Here's how the part is built. I have some questions about the finished solid (model axes, mm). A direction names the side the tool comes from. Round coordinates to 2 decimals unless told otherwise and drop trailing zeros. Write each loop counter-clockwise with the first axis right and the second up, starting at its lowest first coordinate (ties: lowest second). Pieces come first, ordered by that corner, then holes. Notation, with made-up numbers: (-19, -1.5) - (38, -1.5) arc R5 ccw to (38, 6.5) - close; hole circle Ø4 at (-4.75, 65.25). An arc over 180 degrees is marked (long way). Use one line per item in the form item = value. Start each with the question number.
1. I want a section at D-D, the plane z = 6. List the corners of the cut face in (x, y) for me, plus the area to 3 significant figures.
2. Which directions (+Z, -Z, +X, -X, +Y, -Y) give clear straight access to the entire face, cutting with the end or side of a thin tool? Please do faces 1 (the flat face through (-9, 0, 6)), 2 (the cylindrical face through (0, 6, 6)), 3 (the flat face through (8, 5, 4)), 4 (the flat face through (-0.2, -6.5, 12)).
3. Will these pins go through, and if not, where does the flat tip stop? pin 1 (4 mm diameter, centred on y = 8, z = 10, fed in from +X); pin 2 (1.5 mm diameter, centred on x = -7, z = 9.5, fed in from -Y); pin 3 (5 mm diameter, centred on x = -9, z = 6.5, fed in from +Y).
4. We'd pull the mould along Y, two halves only. Please class faces 5 (the cylindrical face through (12.248, 2.845, 5.901)), 6 (the cylindrical face through (-11.17, -10.01, 5.92)), 7 (the cylindrical face through (0, -6, 6)): +Y half, -Y half, draft (parallel to the pull), parting line (faces both ways), or undercut.
5. I want a section at B-B, the plane y = -2. List the corners of the cut face in (x, z) for me, plus the area to 3 significant figures.
6. I want a section at A-A, the plane x = 0. List the corners of the cut face in (y, z) for me, plus the area to 3 significant figures.
7. If I drill on line 1 along X through (y, z) = (4, 4.5); line 2 along X through (y, z) = (-3, 4); line 3 along Z through (x, y) = (10, -6.75), over which ranges is the centre line in solid material (lowest first)?
8. I want a section at C-C, the plane x = 10. List the corners of the cut face in (y, z) for me.
Autodesk Inventor part; units mm, degrees
ref_plane "作業平面1" through (0, 5, 0) normal (0, 1, 0) x (-1, 0, 0)
ref_plane "YZ Plane" through (0, 0, 0) normal (1, 0, 0) x (0, 1, 0)
ref_plane "XY Plane" through (0, 0, 0) normal (0, 0, 1) x (1, 0, 0)
sketch "スケッチ1" plane through (0, 0, 0) normal (0, 0, 1) x (1, 0, 0)
  circle A0 centre (0, 0) radius 15
  circle A1 centre (0, 0) radius 6
  dimension "d0" = 30
  dimension "d1" = 12
extrude "押し出し1" add sketch "スケッチ1" along normal blind 12
sketch "スケッチ2" plane through (0, 0, 0) normal (0, 1, 0) x (-1, 0, 0)
  line L0 (0, 0) -> (0, 12) construction
  line L1 (0, 6) -> (-10, 6) construction
  circle A0 centre (-10, 6) radius 2.25
  line L2 (15, 12) -> (-15, 12) construction
  line L3 (-15, 0) -> (15, 0) construction
  dimension "d4" = 4.5
  dimension "d5" = 10
  dimension "d6" = 6
extrude "押し出し2" cut sketch "スケッチ2" along normal through all both and the other way through all
sketch "スケッチ3" plane through (0, 0, 12) normal (0, 0, 1) x (1, 0, 0)
  line L0 (0, 0) -> (-15.0903, 0) construction
  line L1 (-9, 0.75) -> (21, 0.75)
  line L2 (21, 0.75) -> (21, -0.75)
  line L3 (21, -0.75) -> (-9, -0.75)
  line L4 (-9, -0.75) -> (-9, 0.75)
  line L5 (-9, 0.75) -> (21, -0.75) construction
  line L6 (21, 0.75) -> (-9, -0.75) construction
  point P0 (6, 0)
  dimension "d9" = 9
  dimension "d10" = 1.5
  dimension "d11" = 30
extrude "押し出し3" cut sketch "スケッチ3" against normal through all
ref_plane "作業平面1" through (0, 5, 0) normal (0, 1, 0) x (-1, 0, 0)
sketch "スケッチ4" plane through (0, 5, 0) normal (0, 1, 0) x (-1, 0, 0)
  circle A0 centre (-9.9953, 6) radius 4.5
  line L0 (0, 0) -> (0.0094, 12) construction
  line L1 (15, 12) -> (-14.9812, 12) construction
  line L2 (0.0047, 6) -> (-9.9953, 6) construction
  dimension "d15" = 9
  dimension "d16" = 10
extrude "押し出し4" cut sketch "スケッチ4" along normal through all
properties part number "セットカラー"
Model answer:
q1.outline = (-9, -0.75) - (-9, 0.75) - (-5.95, 0.75) arc R6 cw to (5.95, 0.75) - (7.75, 0.75) - (7.75, 5) - (5.5, 5) - (5.5, 13.96) arc R15 ccw (long way) to (7.75, -12.84) - (7.75, -0.75) - (5.95, -0.75) arc R6 cw to (-5.95, -0.75) - close; (12.25, -8.66) arc R15 ccw to (14.98, -0.75) - (12.25, -0.75) - close; (12.25, 0.75) - (14.98, 0.75) arc R15 ccw to (14.14, 5) - (12.25, 5) - close
q1.area = 460 mm2
q2.face_1 = +Z, -Z, +X
q2.face_2 = +Z, -Z
q2.face_3 = +Y
q2.face_4 = +Z, +X, -X, +Y, -Y
q3.pin_1 = 13.75
q3.pin_2 = -13.64
q3.pin_3 = 13.52
q4.face_5 = draft
q4.face_6 = parting line
q4.face_7 = undercut
q5.outline = (-14.87, 0) - (-5.66, 0) - (-5.66, 12) - (-14.87, 12) - close; (5.66, 0) - (14.87, 0) - (14.87, 12) - (5.66, 12) - close; hole circle Ø4.5 at (10, 6)
q5.area = 205 mm2
q6.outline = (-15, 0) - (-6, 0) - (-6, 12) - (-15, 12) - close; (6, 0) - (15, 0) - (15, 12) - (6, 12) - close
q6.area = 216 mm2
q7.line_1 = -14.46 to -4.47, 4.47 to 8.32, 11.68 to 14.46
q7.line_2 = -14.7 to -5.2, 5.2 to 8.97, 11.03 to 14.7
q7.line_3 = 0 to 3.75, 8.25 to 12
q8.outline = (-11.18, 0) - (-0.75, 0) - (-0.75, 3.75) - (-11.18, 3.75) - close; (-11.18, 8.25) - (-0.75, 8.25) - (-0.75, 12) - (-11.18, 12) - close; (0.75, 0) - (11.18, 0) - (11.18, 1.5) - (5, 1.5) - (5, 3.75) - (0.75, 3.75) - close; (0.75, 8.25) - (5, 8.25) - (5, 10.5) - (11.18, 10.5) - (11.18, 12) - (0.75, 12) - close
